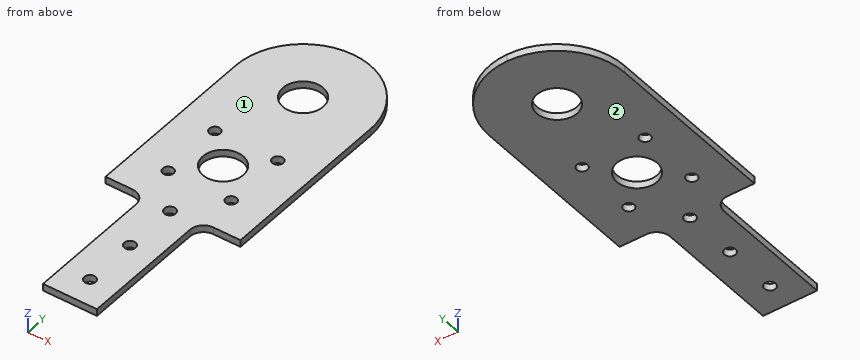
Autodesk Inventor part; units mm, degrees
ref_plane "YZ Plane" through (0, 0, 0) normal (1, 0, 0) x (0, 1, 0)
ref_plane "XZ Plane" through (0, 0, 0) normal (0, 1, 0) x (-1, 0, 0)
ref_plane "XY Plane" through (0, 0, 0) normal (0, 0, 1) x (1, 0, 0)
sketch "Sketch1" plane through (0, 0, 0) normal (0, 0, 1) x (1, 0, 0)
  line L0 (63.5, 1.905) -> (63.5, 128.905)
  line L1 (63.5, 128.905) -> (0, 128.905)
  line L2 (0, 128.905) -> (0, 41.0985)
  circle A0 centre (31.75, 97.155) radius 9.5
  circle A1 centre (31.75, 46.355) radius 9.5
  circle A2 centre (31.75, 12.7) radius 2.6543
  line L3 (19.05, 0) -> (19.05, 14.605)
  line L4 (19.05, 25.4) -> (44.45, 25.4)
  line L5 (44.45, 25.4) -> (44.45, 0)
  line L6 (31.75, 0) -> (31.75, 128.905)
  circle A3 centre (31.75, -12.7) radius 2.6543
  circle A4 centre (31.75, -38.1) radius 2.6543
  line L7 (44.45, 0) -> (44.45, -50.8)
  line L8 (44.45, -50.8) -> (19.05, -50.8)
  line L9 (19.05, -50.8) -> (19.05, 0)
  line L10 (0, 41.0985) -> (0, 27.305)
  line L11 (63.5, 14.605) -> (0, 14.605)
  line L12 (0, 14.605) -> (0, 27.305)
  point P0 (0, 0)
  point P1 (63.5, 27.305)
  point P2 (44.45, 14.605)
  point P3 (31.75, -50.8)
  dimension "d0" = 63.5
  dimension "d1" = 127
  dimension "d3" = 116.205
  dimension "d4" = 31.75
  dimension "d5" = 82.55
  dimension "d12" = 19
  dimension "d13" = 19
  dimension "d14" = 5.3086
  dimension "d29" = 25.4
  dimension "d30" = 25.4
  dimension "d31" = 25.4
  dimension "d32" = 25.4
  dimension "d33" = 50.8
  dimension "d36" = 12.7
extrude "Extrusion1" add sketch "Sketch1" along normal blind 3.302 contours L11 L5 L4 L6 A1 A0 L1 L0 | L11 A2 L6 L4 L5 | L5 L7 L8 L9 L3 L11 A2 | L6 A0 A1 A2 L11 L12 L10 L2 L1
fillet "Fillet1" radius 31.75 1 edges at (63.5, 128.905, 1.651)
fillet "Fillet2" radius 31.75 1 edges at (0, 128.905, 1.651)
sketch "Sketch3" plane through (0, 0, 3.302) normal (0, 0, 1) x (1, 0, 0)
  circle A0 centre (31.75, 46.355) radius 9.5
  circle A1 centre (31.75, 46.355) radius 20.955
  line L0 (31.75, 46.355) -> (4.2793, 73.8257)
  line L1 (4.2793, 73.8257) -> (54.0042, 24.1008)
  line L2 (31.75, 46.355) -> (57.6977, 72.3027)
  line L3 (31.75, 46.355) -> (13.6103, 28.2153)
  line L4 (31.75, 46.355) -> (57.4034, 46.355) construction
  point P0 (0, 0)
  point P1 (46.5674, 61.1724)
  point P2 (46.5674, 31.5376)
  point P3 (16.9326, 61.1724)
  point P4 (16.9326, 31.5376)
  dimension "d16" = 41.91
  dimension "d28" = 135
hole "Hole1" at (46.5674, 61.1724, 3.302) at (46.5674, 31.5376, 3.302) at (16.9326, 61.1724, 3.302) at (16.9326, 31.5376, 3.302) direction (0, 0, -1) diameter 5.1054 depth 16.256 tip angle 118
fillet "Fillet5" radius 6.35 1 edges at (19.05, 14.605, 1.651)
fillet "Fillet6" radius 6.35 1 edges at (44.45, 14.605, 1.651)
equation "\"d13\" = d12"
properties part number "wrist plate 2"
Work out the finished part from the listing and answer in its coordinate system (mm). Face numbers are marked on the shaded views. Give positions to 0.01 mm unless a question says otherwise; leave off trailing zeros. Write each loop counter-clockwise with the first axis right and the second up, starting at its lowest first coordinate (ties: lowest second). Pieces come first, ordered by that corner, then holes.
Q1. Straight lines are drawn through the part: L1, parallel to Y at x = 31.75, z = 1.85 (3 decimals); L2, parallel to Y at x = 31, z = 0.5; L3, parallel to Y at x = 24, z = 1.5. For each, find the intervals that lie inside material, in ascending order.
Answer:
L1: y = -50.8 to -40.754, -35.446 to -15.354, -10.046 to 10.046, 15.354 to 36.855, 55.855 to 87.655, 106.655 to 128.905
L2: y = -50.8 to -40.65, -35.55 to -15.25, -10.15 to 10.15, 15.25 to 36.88, 55.83 to 87.68, 106.63 to 128.9
L3: y = -50.8 to 40.86, 51.85 to 91.66, 102.65 to 127.94
Q2. The part is cut by section B-B on y = 31. Give the vertices of the cut face in (x, z).
Answer:
outline: (0, 0) - (14.44, 0) - (14.44, 3.3) - (0, 3.3) - close; (19.43, 0) - (44.07, 0) - (44.07, 3.3) - (19.43, 3.3) - close; (49.06, 0) - (63.5, 0) - (63.5, 3.3) - (49.06, 3.3) - close
Q3. The part is cut by section D-D on z = 1.5. State how many separate pieces and enclosed holes the cut face has, and give its area (3 significant figures).
Answer:
separate pieces: 1
enclosed holes: 9
area: 7,790 mm2
Q4. For a pull along Z with two mould halves and no side action, classify the marked faces 1 and 2 as released by +Z, released by -Z, zero draft, split by the parting line, or undercut.
Answer:
face 1: released by +Z
face 2: released by -Z
Q5. Given pin 1 (4.5 mm diameter, centred on x = 16.93, y = 61.17, fed in from -Z); pin 2 (1 mm diameter, centred on x = 6.5, z = 1.5, fed in from -Y) (3 decimals); pin 3 (1.7 mm diameter, centred on y = -25, z = 2.5, fed in from -X), each flat-ended and moving along its own axis, determine where each tip first touches the part or whether it passes through.
Answer:
pin 1: passes through
pin 2: stops at y = 14.605
pin 3: stops at x = 19.05
Q6. The part is cut by section C-C on x = 36.5. Give the vertices of the cut face in (y, z).
Answer:
outline: (-50.8, 0) - (38.13, 0) - (38.13, 3.3) - (-50.8, 3.3) - close; (54.58, 0) - (88.93, 0) - (88.93, 3.3) - (54.58, 3.3) - close; (105.38, 0) - (128.55, 0) - (128.55, 3.3) - (105.38, 3.3) - close
Q7. The part is cut by section A-A on y = -38.1. Give the vertices of the cut face in (x, z), and give its area (3 significant figures).
Answer:
outline: (19.05, 0) - (29.1, 0) - (29.1, 3.3) - (19.05, 3.3) - close; (34.4, 0) - (44.45, 0) - (44.45, 3.3) - (34.4, 3.3) - close
area: 66.3 mm2
